from build123d import *

# Parameters (mm, degrees)
SKETCH1_R                    = 4.25
BOSS_EXTRUDE1_DEPTH          = 12.5
BOSS_EXTRUDE4_START          = -3.5
BOSS_EXTRUDE4_DEPTH          = 3.5
CIRPATTERN5_COUNT            = 50
SKETCH5_R                    = 3.75
BOSS_EXTRUDE5_DEPTH          = 3
SKETCH6_R                    = 2.75
BOSS_EXTRUDE6_DEPTH          = 1
SKETCH7_R                    = 2.25
BOSS_EXTRUDE7_DEPTH          = 1.5
SKETCH8_R                    = 2.75
BOSS_EXTRUDE8_DEPTH          = 0.2
SKETCH9_R                    = 2.5
BOSS_EXTRUDE9_DEPTH          = 2
SKETCH10_R                   = 2.75
BOSS_EXTRUDE10_DEPTH         = 0.8
SKETCH11_R                   = 2.55
CUT_EXTRUDE1_DEPTH           = 0.3
SKETCH12_W                   = 4.125233548
SKETCH12_H                   = 0.2
CUT_REVOLVE1_ANGLE           = 6
CUT_REVOLVE1_OTHER_WAY_ANGLE = 6
SKETCH13_W                   = 4.08419342
SKETCH13_H                   = 0.2
CUT_REVOLVE2_ANGLE           = 6
CUT_REVOLVE2_OTHER_WAY_ANGLE = 6
CUT_EXTRUDE2_DEPTH           = 22.995367972
CUT_EXTRUDE2_DEPTH_BACK      = 22.995367972
SKETCH15_R                   = 0.75
SKETCH16_R                   = 3.95
CUT_EXTRUDE3_DEPTH           = 12.2
SKETCH17_R                   = 3.45
CUT_EXTRUDE4_DEPTH           = 3
CUT_EXTRUDE5_REACH           = 18.548
SKETCH19_R                   = 1.95
FILLET1_R                    = 0.2
FILLET2_R                    = 0.15


with BuildPart() as part:
    # Sketch1 → Boss-Extrude1 (new body)
    with BuildSketch(Plane(origin=(0, 0, 0), x_dir=(1, 0, 0), z_dir=(0, 1, 0))):
        with Locations(Location((0, 0, 0), (0, 0, 270))):
            Circle(SKETCH1_R)
    extrude(amount=BOSS_EXTRUDE1_DEPTH)

    # Sketch4 → Boss-Extrude4 (add)
    with BuildSketch(Plane(origin=(0, 12.5, 0), x_dir=(1, 0, 0), z_dir=(0, 1, 0)).offset(BOSS_EXTRUDE4_START)):
        with BuildLine():
            ThreePointArc((-4.233011765, 0.379620073), (-4.25, 0), (-4.233011765, -0.379620073))
            ThreePointArc((-4.233011765, -0.379620073), (-4.63, 0), (-4.233011765, 0.379620073))
        make_face()
    boss_extrude4 = extrude(amount=BOSS_EXTRUDE4_DEPTH)

    # CirPattern5: Boss-Extrude4 ×50 about axis
    cirpattern5_axis = Axis((0, 0, 0), (0, 1, 0))
    for i in range(1, CIRPATTERN5_COUNT):
        add(boss_extrude4.rotate(cirpattern5_axis, i * 360 / CIRPATTERN5_COUNT))

    # Sketch5 → Boss-Extrude5 (add)
    with BuildSketch(Plane(origin=(0, 12.5, 0), x_dir=(1, 0, 0), z_dir=(0, 1, 0))):
        with Locations(Location((0, 0, 0), (0, 0, 270))):
            Circle(SKETCH5_R)
    extrude(amount=BOSS_EXTRUDE5_DEPTH)

    # Sketch6 → Boss-Extrude6 (add)
    with BuildSketch(Plane(origin=(0, 15.5, 0), x_dir=(1, 0, 0), z_dir=(0, 1, 0))):
        with Locations(Location((0, 0, 0), (0, 0, 270))):
            Circle(SKETCH6_R)
    extrude(amount=BOSS_EXTRUDE6_DEPTH)

    # Sketch7 → Boss-Extrude7 (add)
    with BuildSketch(Plane(origin=(0, 16.5, 0), x_dir=(1, 0, 0), z_dir=(0, 1, 0))):
        with Locations(Location((0, 0, 0), (0, 0, 270))):
            Circle(SKETCH7_R)
    extrude(amount=BOSS_EXTRUDE7_DEPTH)

    # Sketch8 → Boss-Extrude8 (add)
    with BuildSketch(Plane(origin=(0, 18, 0), x_dir=(1, 0, 0), z_dir=(0, 1, 0))):
        with Locations(Location((0, 0, 0), (0, 0, 270))):
            Circle(SKETCH8_R)
    extrude(amount=BOSS_EXTRUDE8_DEPTH)

    # Sketch9 → Boss-Extrude9 (add)
    with BuildSketch(Plane(origin=(0, 18.2, 0), x_dir=(1, 0, 0), z_dir=(0, 1, 0))):
        with Locations(Location((0, 0, 0), (0, 0, 270))):
            Circle(SKETCH9_R)
    extrude(amount=BOSS_EXTRUDE9_DEPTH)

    # Sketch10 → Boss-Extrude10 (add)
    with BuildSketch(Plane(origin=(0, 20.2, 0), x_dir=(1, 0, 0), z_dir=(0, 1, 0))):
        with Locations(Location((0, 0, 0), (0, 0, 270))):
            Circle(SKETCH10_R)
    extrude(amount=BOSS_EXTRUDE10_DEPTH)

    # Sketch11 → Cut-Extrude1 (cut)
    with BuildSketch(Plane(origin=(0, 21, 0), x_dir=(1, 0, 0), z_dir=(0, 1, 0))):
        with Locations(Location((0, 0, 0), (0, 0, 270))):
            Circle(SKETCH11_R)
    extrude(amount=-CUT_EXTRUDE1_DEPTH, mode=Mode.SUBTRACT)

    # Sketch12 → Cut-Revolve1 (revolve, cut)
    with BuildSketch(Plane(origin=(0, 20.7, 0), x_dir=(1, 0, 0), z_dir=(0, 1, 0))):
        with Locations((-0.862616774, -1.1)):
            Rectangle(SKETCH12_W, SKETCH12_H)
    revolve(axis=Axis((1.2, 20.7, -2.474368606), (0, 0, 1)), revolution_arc=CUT_REVOLVE1_ANGLE, mode=Mode.SUBTRACT)

    # Sketch12 → Cut-Revolve1 other way (revolve, cut)
    with BuildSketch(Plane(origin=(0, 20.7, 0), x_dir=(1, 0, 0), z_dir=(0, 1, 0))):
        with Locations((-0.862616774, -1.1)):
            Rectangle(SKETCH12_W, SKETCH12_H)
    revolve(axis=Axis((1.2, 20.7, -2.474368606), (0, 0, -1)), revolution_arc=CUT_REVOLVE1_OTHER_WAY_ANGLE, mode=Mode.SUBTRACT)

    # Sketch13 → Cut-Revolve2 (revolve, cut)
    with BuildSketch(Plane(origin=(0, 20.7, 0), x_dir=(1, 0, 0), z_dir=(0, 1, 0))):
        with Locations((0.84209671, 1.1)):
            Rectangle(SKETCH13_W, SKETCH13_H)
    revolve(axis=Axis((-1.2, 20.7, -2.950120445), (0, 0, 1)), revolution_arc=CUT_REVOLVE2_ANGLE, mode=Mode.SUBTRACT)

    # Sketch13 → Cut-Revolve2 other way (revolve, cut)
    with BuildSketch(Plane(origin=(0, 20.7, 0), x_dir=(1, 0, 0), z_dir=(0, 1, 0))):
        with Locations((0.84209671, 1.1)):
            Rectangle(SKETCH13_W, SKETCH13_H)
    revolve(axis=Axis((-1.2, 20.7, -2.950120445), (0, 0, -1)), revolution_arc=CUT_REVOLVE2_OTHER_WAY_ANGLE, mode=Mode.SUBTRACT)

    # Sketch15 → Cut-Extrude2 (cut, two sides: drawn at the far end of the back side and taken through both)
    with BuildSketch(Plane.XY.offset(-CUT_EXTRUDE2_DEPTH_BACK)):
        with Locations(Location((0, 19.270988454, 0), (0, 0, 89.999999982))):
            Circle(SKETCH15_R)
    extrude(amount=CUT_EXTRUDE2_DEPTH + CUT_EXTRUDE2_DEPTH_BACK, mode=Mode.SUBTRACT)

    # Sketch16 → Cut-Extrude3 (cut)
    with BuildSketch(Plane.XZ):
        with Locations(Location((0, 0, 0), (0, 0, 270))):
            Circle(SKETCH16_R)
    extrude(amount=-CUT_EXTRUDE3_DEPTH, mode=Mode.SUBTRACT)

    # Sketch17 → Cut-Extrude4 (cut)
    with BuildSketch(Plane.XZ.offset(-12.2)):
        with Locations(Location((0, 0, 0), (0, 0, 270))):
            Circle(SKETCH17_R)
    extrude(amount=-CUT_EXTRUDE4_DEPTH, mode=Mode.SUBTRACT)

    # Cut-Extrude5: up to this face of the body (flat: up to its plane)
    cut_extrude5_end = Plane(part.part.faces().sort_by_distance((0, 20.2, -2.672218254))[0])
    # Sketch19 → Cut-Extrude5 (cut, up to the picked face)
    with BuildSketch(Plane.XZ.offset(-15.2), mode=Mode.PRIVATE) as cut_extrude5_sk1:
        with Locations(Location((0, 0, 0), (0, 0, 270))):
            Circle(SKETCH19_R)
    cut_extrude5_tool1 = split(extrude(cut_extrude5_sk1.sketch, amount=-CUT_EXTRUDE5_REACH, mode=Mode.PRIVATE), bisect_by=cut_extrude5_end, keep=Keep.BOTH, mode=Mode.PRIVATE)
    add(cut_extrude5_tool1.solids().sort_by(Axis((0, 15.2, 0), (0, 1, 0)))[0], mode=Mode.SUBTRACT)

    # Fillet1
    fillet1_edges = [part.edges().sort_by_distance(p)[0] for p in [
        (0, 16.5, -2.25),
        (0, 18, -2.25),
    ]]
    fillet(fillet1_edges, radius=FILLET1_R)

    # Fillet2
    fillet2_edges = [part.edges().sort_by_distance(p)[0] for p in [
        (0, 0, -4.25),
        (0, 0, 3.95),
    ]]
    fillet(fillet2_edges, radius=FILLET2_R - 0.0001)  # a hair under: the kernel refuses the full size


solid = part.part
Verification items for the finished model (mm, model axes). A direction names the side the tool comes from. Give positions to 0.01 mm unless a question says otherwise; leave off trailing zeros. Loops run counter-clockwise (first coordinate to the right, second up) from the corner with the lowest first, then second, coordinate; pieces in that order, holes last.
1) Draft check along X on faces 1 (the flat face through (-4, 12.5, 0)), 2 (the cylindrical face through (0.732, 19.108, -2.155)), 3 (the cylindrical face through (-2.685, 15.993, -0.596)). Enter one of: pulls with the +X half, pulls with the -X half, needs draft (parallel to the pull), parting line crosses it, or undercut.
2) Set-up check for faces 4 (the flat face through (0, 20.7, 0)), 5 (the cylindrical face through (-0.96, 19.19, 2.31)), 6 (the cylindrical face through (0.732, 19.108, 2.145)), 7 (the flat face through (0, 20.2, 0)): record each of +Z, -Z, +X, -X, +Y, -Y from which the full face is reachable in a straight line by a thin tool's end or side.
3) Thickness scan on line 1 along X through (y, z) = (14.25, 0); line 2 along X through (y, z) = (16.35, 0); line 3 along Y through (x, z) = (-0.5, -2.25). Record the ranges inside material, lowest first.
4) Depth check by flat-ended pin: pin 1 Ø1 at (y, z) = (12.5, 3) entering from -X; pin 2 Ø1.6 at (x, z) = (1, -1) entering from -Y; pin 3 Ø1 at (x, y) = (0, 5) entering from -Z. Enter the tip coordinate at first touch or a pass-through.
5) Sectioned sample at A-A, the plane y = 6. Enter the section's corners in (x, z).
Answers:
1. face 1: needs draft
1. face 2: undercut
1. face 3: parting line crosses it
2. face 4: +Y
2. face 5: none
2. face 6: +Z, -Z
2. face 7: -Y
3. line 1: x = -3.75 to -3.45, 3.45 to 3.75
3. line 2: x = -2.75 to -1.95, 1.95 to 2.75
3. line 3: y = 15.2 to 16.56, 17.94 to 18.71, 19.83 to 20.7
4. pin 1: stops at x = -3.82
4. pin 2: stops at y = 15.2
4. pin 3: stops at z = -4.25
5. outline: circle Ø8.5 at (0, 0); hole circle Ø7.9 at (0, 0)
